Can you work these out from the drawing? Everything is in mm from the part's minimum corner. Round coordinates to 2 decimals unless told otherwise and drop trailing zeros. Order: outer loops, then holes, each group sorted by start corner. A loop starts at its lowest first (then second) coordinate and runs counter-clockwise, first axis right, second up. Notation, with made-up numbers: (70.5, 2.25) -> (75.5, 2.25) arc R6 ccw to (75.5, 10.25) -> close; hole circle Ø6 at (-10, -32.75). An arc over 180 degrees is marked (long way). One line per item, written item: value.
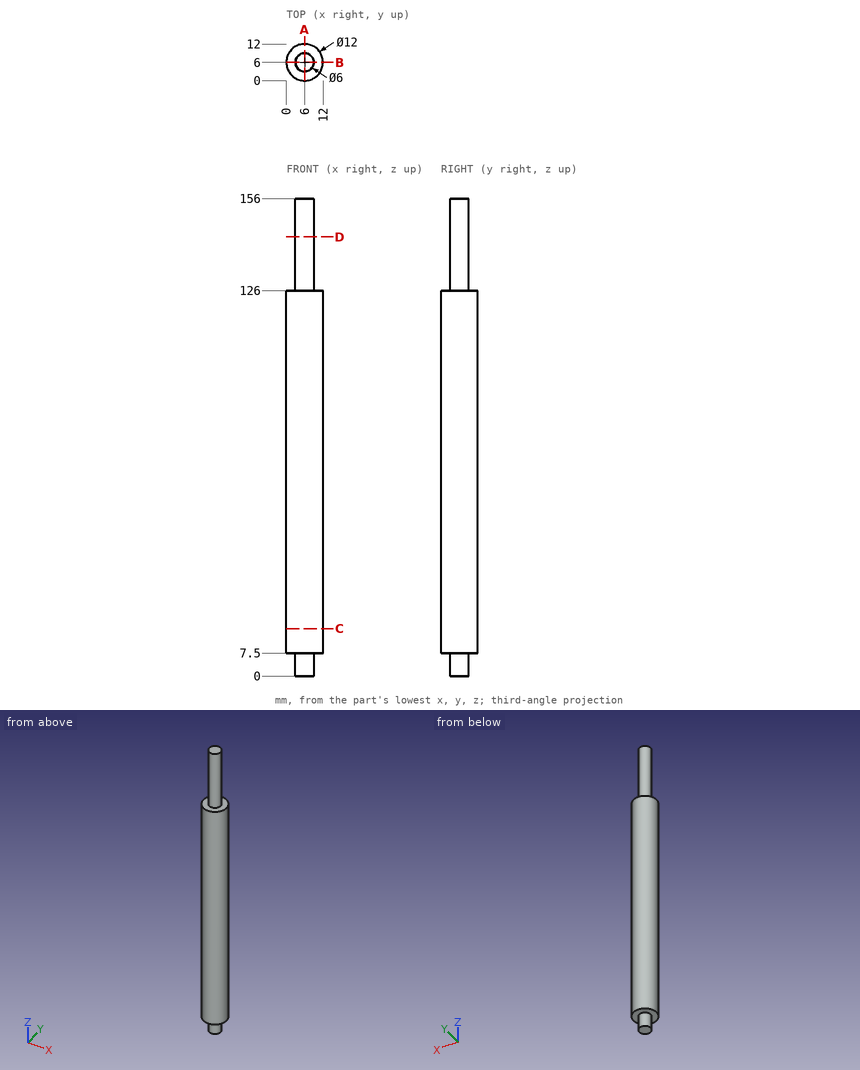
Q1. I want a section at C-C on z = 15.5. Write out the boundary of the cut face in (x, y).
Answers:
outline: circle Ø12 at (6, 6)
Q2. I need wall thicknesses on line 1 along Z through (x, y) = (3.5, 10); line 2 along Y through (x, z) = (6.25, 24.5); line 3 along Y through (x, z) = (8.25, 77). Which ranges of each line are inside material? Lowest first, please.
Answers:
line 1: 7.5 to 126
line 2: 0.01 to 11.99
line 3: 0.44 to 11.56
Q3. I want a section at A-A on x = 6. Write out the boundary of the cut face in (y, z), then the cut area to 3 significant figures.
Answers:
outline: (0, 7.5) -> (3, 7.5) -> (3, 0) -> (9, 0) -> (9, 7.5) -> (12, 7.5) -> (12, 126) -> (9, 126) -> (9, 156) -> (3, 156) -> (3, 126) -> (0, 126) -> close
area: 1,650 mm2
Q4. For P1, Ø1.5, axis at y = 3, z = 130.5, coming from the +X side; P2, Ø4, axis at x = 9.5, z = 131, coming from the -Y side; P3, Ø1.5, axis at x = 2, z = 54.5, coming from the +Y side, each with a flat end and sliding along its axis, tell me the tip position at first contact or that it passes through.
Answers:
P1: x = 7.98
P2: y = 3.4
P3: y = 11.04
Q5. I want a section at D-D on z = 143.5. Write out the boundary of the cut face in (x, y), then the cut area to 3 significant figures.
Answers:
outline: circle Ø6 at (6, 6)
area: 28.3 mm2
